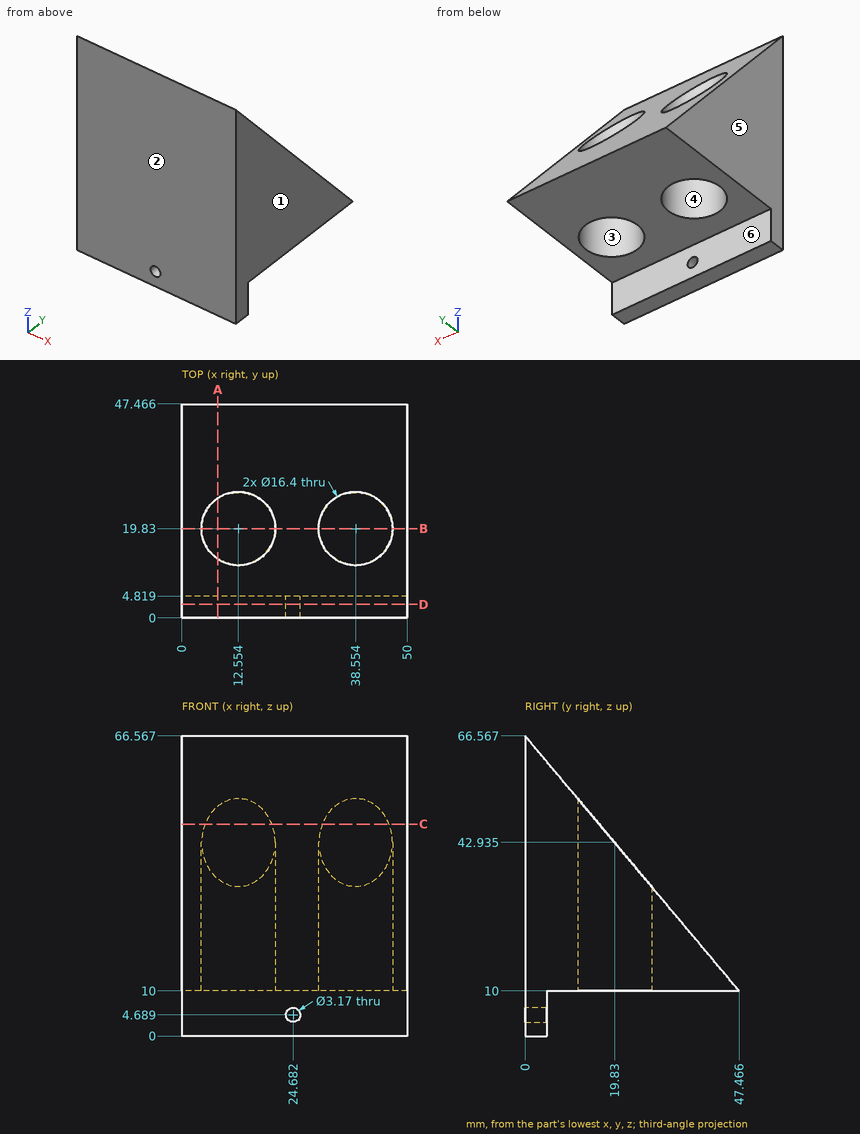
Answer from the drawing. Dimensions are ordinates in mm from the lowest x, y and z of the part. A direction names the side the tool comes from. Round coordinates to 2 decimals unless told otherwise and drop trailing zeros. Write each loop counter-clockwise with the first axis right and the second up, starting at its lowest first coordinate (ties: lowest second). Pieces come first, ordered by that corner, then holes.
1. The part is cut by section C-C, the plane z = 47. Determine the outline of the cut face in (x, y) (1 decimal).
2. Given pin 1 Ø5 at (x, y) = (15, 31) entering from +Z; pin 2 Ø12 at (x, z) = (36, 46.5) entering from +Y (1 decimal); pin 3 Ø21.5 at (x, y) = (35, 19.5) entering from -Z, each flat-ended and moving along its own axis, determine where each tip first touches the part or whether it passes through.
3. The part is cut by section D-D, the plane y = 3. Determine the outline of the cut face in (x, z) (1 decimal), then the cut area to 3 significant figures.
4. The part is cut by section B-B, the plane y = 19.83. Determine the outline of the cut face in (x, z) (1 decimal).
5. Straight lines are drawn through the part: L1, parallel to X at y = 19.5, z = 17; L2, parallel to X at y = 19.83, z = 36.5 (1 decimal); L3, parallel to Y at x = 45, z = 15. For each, find the intervals that lie inside material, in ascending order.
6. Determine the mould class of the marked faces 1, 2, 3 and 4 for opening direction Y: pulls with the +Y half, pulls with the -Y half, needs draft (parallel to the pull), parting line crosses it, or undercut.
7. The part is cut by section A-A, the plane x = 8. Determine the outline of the cut face in (y, z) (1 decimal).
8. Which of the six approach directions +Z, -Z, +X, -X, +Y, -Y give full straight-line access (tool end or side, diameter ignored) to the marked faces 5 and 6?
Values:
1. outline: (0, 0) - (50, 0) - (50, 16.4) - (46, 16.4) arc R8.2 cw to (31.1, 16.4) - (20, 16.4) arc R8.2 cw to (5.1, 16.4) - (0, 16.4) - close
2. pin 1: stops at z = 32.6
2. pin 2: stops at y = 18.7
2. pin 3: stops at z = 10
3. outline: (0, 0) - (50, 0) - (50, 63) - (0, 63) - close; hole circle Ø3.2 at (24.7, 4.7)
3. area: 3,140 mm2
4. outline: (0, 10) - (4.4, 10) - (4.4, 42.9) - (0, 42.9) - close; (20.8, 10) - (30.4, 10) - (30.4, 42.9) - (20.8, 42.9) - close; (46.8, 10) - (50, 10) - (50, 42.9) - (46.8, 42.9) - close
5. L1: x = 0 to 4.36, 20.75 to 30.36, 46.75 to 50
5. L2: x = 0 to 4.4, 20.8 to 30.4, 46.8 to 50
5. L3: y = 0 to 14.76, 24.9 to 43.27
6. face 1: needs draft
6. face 2: pulls with the -Y half
6. face 3: undercut
6. face 4: undercut
7. outline: (0, 0) - (4.8, 0) - (4.8, 10) - (13, 10) - (13, 51.1) - (0, 66.6) - close; (26.6, 10) - (47.5, 10) - (26.6, 34.8) - close
8. face 5: +Z, -Z, -X, +Y, -Y
8. face 6: -Z, +X, -X, +Y
